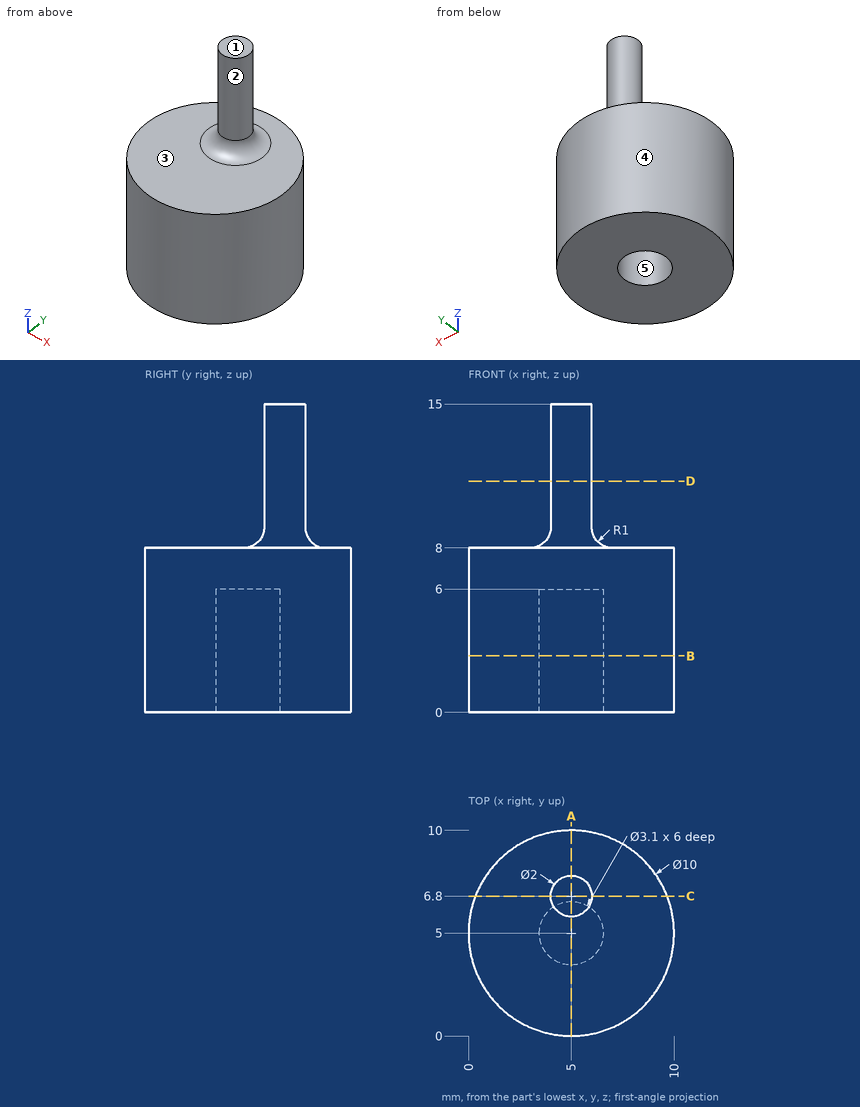
Here's the drawing with two shaded views (mm, measured from the low corner). I have some questions. A direction names the side the tool comes from. Give positions to 0.01 mm unless a question says otherwise; leave off trailing zeros. Order: outer loops, then holes, each group sorted by start corner. A loop starts at its lowest first (then second) coordinate and runs counter-clockwise, first axis right, second up. Notation, with made-up numbers: M -17,-1.5 L 9,-1.5 A21 cw 9,22.5 Z; hole C -8,11 d2. An arc over 180 degrees is marked long. Answer as a JSON object with one key per item and string values. Group by question number.
1) Please list where these lines run through material, in increasing order: L1, parallel to Y at x = 5, z = 2.6; L2, parallel to Z at x = 8, y = 5.25; L3, parallel to Z at x = 4.5, y = 3.75. Write a range as [from, to].
2) Suppose I cut it at A-A, the plane x = 5. Write out the boundary of the cut face in (y, z).
3) Suppose I cut it at D-D, the plane z = 11.25. Write out the boundary of the cut face in (x, y), plus the area to 3 significant figures.
4) Suppose I cut it at C-C, the plane y = 6.8. Write out the boundary of the cut face in (x, z), plus the area to 3 significant figures.
5) On a 3-axis mill with a long thin cutter (end or side, diameter ignored), from which of +Z, -Z, +X, -X, +Y, -Y can I reach the whole of each face in a straight line? I mean the marked faces 1 and 2. Say none if no direction works.
6) We'd pull the mould along Y, two halves only. Please class the marked faces 3, 4 and 5: pulls with the +Y half, pulls with the -Y half, needs draft (parallel to the pull), parting line crosses it, or undercut.
7) I'm going to push flat-ended pins straight in: pin 1 Ø6 at (x, z) = (5, 12.5) entering from -Y; pin 2 Ø2 at (y, z) = (6, 11) entering from +X; pin 3 Ø1 at (x, z) = (1, 5.5) entering from +Y; pin 4 Ø3.5 at (x, y) = (5.5, 5) entering from -Z. Where does each tip first touch, or does it pass through?
8) Suppose I cut it at B-B, the plane z = 2.75. Write out the boundary of the cut face in (x, y), plus the area to 3 significant figures.
Results found:
{
 "1": {"L1": "[0, 3.45], [6.55, 10]", "L2": "[0, 8]", "L3": "[6, 8]"},
 "2": {"outline": "M 0,0 L 3.45,0 L 3.45,6 L 6.55,6 L 6.55,0 L 10,0 L 10,8 L 8.8,8 A1 cw 7.8,9 L 7.8,15 L 5.8,15 L 5.8,9 A1 cw 4.8,8 L 0,8 Z"},
 "3": {"outline": "C 5,6.8 d2", "area": "3.14 mm²"},
 "4": {"outline": "M 0.34,0 L 9.66,0 L 9.66,8 L 7,8 A1 cw 6,9 L 6,15 L 4,15 L 4,9 A1 cw 3,8 L 0.34,8 Z", "area": "89.1 mm²"},
 "5": {"face 1": "+Z, +X, -X, +Y, -Y", "face 2": "+Z"},
 "6": {"face 3": "needs draft", "face 4": "parting line crosses it", "face 5": "undercut"},
 "7": {"pin 1": "y = 5.8", "pin 2": "x = 6", "pin 3": "y = 8.57", "pin 4": "z = 0"},
 "8": {"outline": "C 5,5 d10; hole C 5,5 d3.1", "area": "71.0 mm²"}
}
